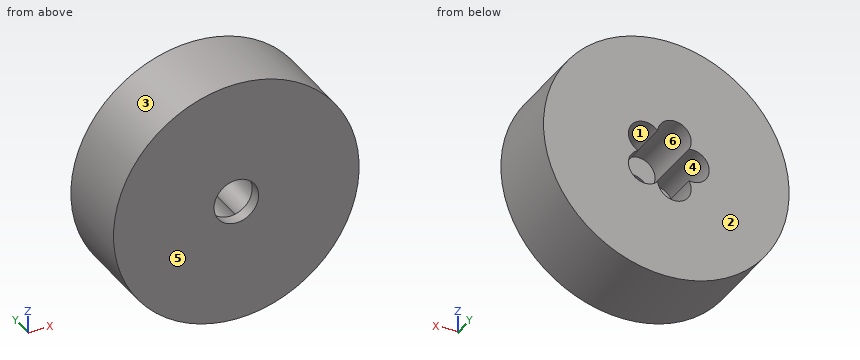
```python
from build123d import *

# Parameters (mm, degrees)
SKETCH1_R           = 27.5
BOSS_EXTRUDE1_DEPTH = 18
SKETCH2_R           = 5
CUT_EXTRUDE1_DEPTH  = 43.854404674
SKETCH3_R           = 3.769575295
CUT_EXTRUDE2_DEPTH  = 15.258815
CIRPATTERN1_START   = 2.741185271
CIRPATTERN1_DEPTH   = 15.258814729


# Read off the part's stored shape, not the designer's step: CirPattern1
with BuildPart() as part:
    # Sketch1 → Boss-Extrude1 (new body)
    with BuildSketch(Plane(origin=(0, 0, 0), x_dir=(1, 0, 0), z_dir=(0, 1, 0))):
        with Locations(Location((0, 0, 0), (0, 0, 270))):
            Circle(SKETCH1_R)
    extrude(amount=BOSS_EXTRUDE1_DEPTH)

    # Sketch2 → Cut-Extrude1 (cut, through all)
    with BuildSketch(Plane(origin=(0, 0, 0), x_dir=(1, 0, 0), z_dir=(0, 1, 0))):
        with Locations(Location((0, 0, 0), (0, 0, 270))):
            Circle(SKETCH2_R)
    extrude(amount=CUT_EXTRUDE1_DEPTH, mode=Mode.SUBTRACT)

    # Sketch3 → Cut-Extrude2 (cut)
    with BuildSketch(Plane(origin=(0, 18, 0), x_dir=(1, 0, 0), z_dir=(0, 1, 0))):
        with Locations((-5.832726886, 0)):
            Circle(SKETCH3_R)
    extrude(amount=-CUT_EXTRUDE2_DEPTH, mode=Mode.SUBTRACT)

    # CirPattern1 outline → CirPattern1 (cut)
    with BuildSketch(Plane(origin=(0, 0, 0), x_dir=(1, 0, 0), z_dir=(0, 1, 0)).offset(CIRPATTERN1_START)):
        with BuildLine():
            ThreePointArc((-3.841342643, -3.200638483), (-4.441257242, -3.50335698), (-5.085388027, -3.694750673))
            ThreePointArc((-5.085388027, -3.694750673), (-2.967274559, -9.132332061), (1.94244538, -5.978232169))
            ThreePointArc((1.94244538, -5.978232169), (7.76842565, -5.64409161), (6.285885293, 0))
            ThreePointArc((6.285885293, 0), (7.76842565, 5.64409161), (1.94244538, 5.978232169))
            ThreePointArc((1.94244538, 5.978232169), (-2.967274559, 9.132332061), (-5.085388027, 3.694750673))
            ThreePointArc((-5.085388027, 3.694750673), (-4.441257242, 3.50335698), (-3.841342643, 3.200638483))
            ThreePointArc((-3.841342643, 3.200638483), (5, 0), (-3.841342643, -3.200638483))
        make_face()
    extrude(amount=CIRPATTERN1_DEPTH, mode=Mode.SUBTRACT)


solid = part.part
```
The listing builds one solid part. Answer for the finished solid, in the listing's coordinates (mm). Face numbers are marked on the shaded views. A direction names the side the tool comes from. Give positions to 0.01 mm unless a question says otherwise; leave off trailing zeros. Order: outer loops, then holes, each group sorted by start corner. A loop starts at its lowest first (then second) coordinate and runs counter-clockwise, first axis right, second up.
Item 1: For a pull along X with two mould halves and no side action, classify the marked faces 3, 4, 5 and 6 as pulls with the +X half, pulls with the -X half, needs draft (parallel to the pull), parting line crosses it, or undercut.
From the geometry:
face 3: parting line crosses it
face 4: undercut
face 5: needs draft
face 6: undercut
Item 2: The part is cut by section A-A, the plane x = 3.5. Give the vertices of the cut face in (y, z).
From the geometry:
outline: (0, -27.28) - (18, -27.28) - (18, -7) - (2.74, -7) - (2.74, -3.57) - (0, -3.57) - close; (0, 3.57) - (2.74, 3.57) - (2.74, 7) - (18, 7) - (18, 27.28) - (0, 27.28) - close
Item 3: The part is cut by section B-B, the plane y = 17. Give the vertices of the cut face in (x, z).
From the geometry:
outline: circle Ø55 at (0, 0); hole (-5.09, -3.69) arc R3.77 ccw (long way) to (1.94, -5.98) arc R3.77 ccw (long way) to (6.29, 0) arc R3.77 ccw (long way) to (1.94, 5.98) arc R3.77 ccw (long way) to (-5.09, 3.69) arc R3.77 ccw (long way) to start
Item 4: Given pin 1 Ø4.5 at (x, z) = (-1.8, 5.55) entering from +Y; pin 2 Ø10 at (y, z) = (11.5, 18.5) entering from +X; pin 3 Ø10 at (x, y) = (20, 7) entering from -Z, each flat-ended and moving along its own axis, determine where each tip first touches the part or whether it passes through.
From the geometry:
pin 1: stops at y = 2.74
pin 2: stops at x = 23.96
pin 3: stops at z = -23.05
Item 5: The part is cut by section D-D, the plane x = -18.5. Give the vertices of the cut face in (y, z), and give its area (3 significant figures).
From the geometry:
outline: (0, -20.35) - (18, -20.35) - (18, 20.35) - (0, 20.35) - close
area: 732 mm2
Item 6: The part is cut by section C-C, the plane z = 21. Give the vertices of the cut face in (x, y), and give its area (3 significant figures).
From the geometry:
outline: (-17.76, 0) - (17.76, 0) - (17.76, 18) - (-17.76, 18) - close
area: 639 mm2
Item 7: Which of the six approach directions +Z, -Z, +X, -X, +Y, -Y give full straight-line access (tool end or side, diameter ignored) to the marked faces 1 and 2?
From the geometry:
face 1: +Y
face 2: +Z, -Z, +X, -X, +Y
Item 8: Find the intervals of material crossed by probe 1 along X at (y, z) = (1.5, -3); probe 2 along Y at (x, z) = (-1, -8); probe 3 along X at (y, z) = (14.5, 9), in increasing order.
From the geometry:
probe 1: x = -27.34 to -4, 4 to 27.34
probe 2: y = 0 to 2.74
probe 3: x = -25.99 to -3.32, -0.29 to 25.99
